from build123d import *

# Parameters (mm, degrees)
SKETCH_1_R          = 2.5
EXTRUDE_1_DEPTH     = 1.5
SKETCH_2_R          = 1.5
EXTRUDE_2_DEPTH     = 25
SKETCH_3_R          = 0.8
CUT_EXTRUDE_1_DEPTH = 27.916537667
CHAMFER_1_SIZE      = 0.5


with BuildPart() as part:
    # 草图1 → 凸台-拉伸1 (new body)
    with BuildSketch(Plane.XY):
        Circle(SKETCH_1_R)
    extrude(amount=EXTRUDE_1_DEPTH)

    # 草图2 → 凸台-拉伸2 (add)
    with BuildSketch(Plane.XY.offset(1.5)):
        Circle(SKETCH_2_R)
    extrude(amount=EXTRUDE_2_DEPTH)

    # 草图3 → 切除-拉伸1 (cut, through all)
    with BuildSketch(Plane(origin=(1.5, 0, 0), x_dir=(0, 0, -1), z_dir=(1, 0, 0))):
        with Locations(Location((-24.5, 0, 0), (0, 0, 180))):
            Circle(SKETCH_3_R)
    extrude(amount=-CUT_EXTRUDE_1_DEPTH, mode=Mode.SUBTRACT)

    # 倒角1
    chamfer_1_edges = [part.edges().sort_by_distance(p)[0] for p in [
        (-1.5, 0, 26.5),
    ]]
    chamfer(chamfer_1_edges, length=CHAMFER_1_SIZE)


solid = part.part
Source: CAD feature listing. Evaluate the final solid. Frame: model axes, mm. A direction names the side the tool comes from. Coordinates: 2 decimals unless noted, no trailing zeros. Loops run counter-clockwise (first coordinate to the right, second up) from the corner with the lowest first, then second, coordinate; pieces in that order, holes last. Notation, with made-up numbers: (69.25, -10.75) - (113.25, -10.75) arc R5 ccw to (113.25, -5.75) - close; hole circle Ø11 at (36, -36). An arc over 180 degrees is marked (long way). One line per question, with ' | ' between items.
1) Section A-A, the plane y = 0. Return loops of the section in (x, z).
Report:
outline: (-2.5, 0) - (2.5, 0) - (2.5, 1.5) - (1.5, 1.5) - (1.5, 23.7) - (-1.5, 23.7) - (-1.5, 1.5) - (-2.5, 1.5) - close; (-1.5, 25.3) - (1.5, 25.3) - (1.5, 26) - (1, 26.5) - (-1, 26.5) - (-1.5, 26) - close
2) Section C-C, the plane z = 20. Return loops of the section in (x, y).
Report:
outline: circle Ø3 at (0, 0)
3) Set-up query: faces 1 (the face through (0, -2, 1.5)), 2 (the face through (0, 0, 26.5)). Return all of +Z, -Z, +X, -X, +Y, -Y with unobstructed straight access to the full face (end or side cutting, diameter ignored); none if empty.
Report:
face 1: +Z | face 2: +Z, +X, -X, +Y, -Y
4) Pull-direction query (Y, two-part tool) for faces 3 (the face through (0, 0, 0)), 4 (the face through (-0.54, -2.44, 0.74)), 5 (the face through (0, 0, 23.7)); classes: released by +Y, released by -Y, zero draft, split by the parting line, or undercut.
Report:
face 3: zero draft | face 4: split by the parting line | face 5: undercut
5) Section B-B, the plane x = 0. Return loops of the section in (y, z).
Report:
outline: (-2.5, 0) - (2.5, 0) - (2.5, 1.5) - (1.5, 1.5) - (1.5, 26) - (1, 26.5) - (-1, 26.5) - (-1.5, 26) - (-1.5, 1.5) - (-2.5, 1.5) - close; hole circle Ø1.6 at (0, 24.5)
6) Section D-D, the plane z = 24.5. Return loops of the section in (x, y).
Report:
outline: (-1.27, -0.8) arc R1.5 ccw to (1.27, -0.8) - close; (-1.27, 0.8) - (1.27, 0.8) arc R1.5 ccw to start
7) Line query: line 1 along Y through (x, z) = (0.1, 24.5); line 2 along Z through (x, y) = (0.8, -1.5); line 3 along Y through (x, z) = (0.4, 24.5). Output: solid intervals per line, ascending.
Report:
line 1: y = -1.5 to -0.8, 0.8 to 1.5 | line 2: z = 0 to 1.5 | line 3: y = -1.45 to -0.8, 0.8 to 1.45
8) First-contact query: P1, Ø1.5, axis at x = -0.5, y = -1, coming from the +Z side. Flat tip, straight axial feed; report the tip coordinate or a pass-through.
Report:
P1: stops at z = 26.5
